Input: part model. Units: mm. Frame: model coordinates. A direction names the side the tool comes from. Give positions to 0.01 mm unless a question says otherwise; leave off trailing zeros. Loops run counter-clockwise (first coordinate to the right, second up) from the corner with the lowest first, then second, coordinate; pieces in that order, holes last. Notation, with made-up numbers: (-30, 7.5) - (12, 7.5) arc R28 ccw to (12, 37.5) - close; hole circle Ø1 at (-7, 6.5). An arc over 180 degrees is marked (long way). Answer as a JSON object with one key per item and string values.
Autodesk Inventor part; units mm, degrees
ref_plane "YZ Plane" through (0, 0, 0) normal (1, 0, 0) x (0, 1, 0)
ref_plane "XZ Plane" through (0, 0, 0) normal (0, 1, 0) x (-1, 0, 0)
ref_plane "XY Plane" through (0, 0, 0) normal (0, 0, 1) x (1, 0, 0)
sketch "Sketch1" plane through (0, 0, 0) normal (1, 0, 0) x (0, 1, 0)
  circle A0 centre (0, 0) radius 35
  line L0 (29.5804, -5) -> (4.8166, -1.3417)
  line L1 (36.6755, 0) -> (35, 0)
  line L2 (29.5804, 5) -> (4.8166, 1.3417)
  line L3 (17.381, 24.452) -> (2.4572, 4.3546)
  line L4 (24.452, 17.381) -> (4.3546, 2.4572)
  line L5 (-5, 29.5804) -> (-1.3417, 4.8166)
  line L6 (5, 29.5804) -> (1.3417, 4.8166)
  line L7 (-24.452, 17.381) -> (-4.3546, 2.4572)
  line L8 (-17.381, 24.452) -> (-2.4572, 4.3546)
  line L9 (-29.5804, -5) -> (-4.8166, -1.3417)
  line L10 (-29.5804, 5) -> (-4.8166, 1.3417)
  line L11 (-17.381, -24.452) -> (-2.4572, -4.3546)
  line L12 (-24.452, -17.381) -> (-4.3546, -2.4572)
  line L13 (5, -29.5804) -> (1.3417, -4.8166)
  line L14 (-5, -29.5804) -> (-1.3417, -4.8166)
  line L15 (24.452, -17.381) -> (4.3546, -2.4572)
  line L16 (17.381, -24.452) -> (2.4572, -4.3546)
  arc A1 (4.8166, 1.3417) -> (4.3546, 2.4572) centre (0, 0) ccw
  arc A2 (2.4572, 4.3546) -> (1.3417, 4.8166) centre (0, 0) ccw
  arc A3 (-1.3417, 4.8166) -> (-2.4572, 4.3546) centre (0, 0) ccw
  arc A4 (-4.3546, 2.4572) -> (-4.8166, 1.3417) centre (0, 0) ccw
  arc A5 (-4.8166, -1.3417) -> (-4.3546, -2.4572) centre (0, 0) ccw
  arc A6 (-2.4572, -4.3546) -> (-1.3417, -4.8166) centre (0, 0) ccw
  arc A7 (1.3417, -4.8166) -> (2.4572, -4.3546) centre (0, 0) ccw
  arc A8 (4.3546, -2.4572) -> (4.8166, -1.3417) centre (0, 0) ccw
  arc A9 (29.5804, 5) -> (24.452, 17.381) centre (0, 0) ccw
  arc A10 (24.452, -17.381) -> (29.5804, -5) centre (0, 0) ccw
  arc A11 (5, -29.5804) -> (17.381, -24.452) centre (0, 0) ccw
  arc A12 (-17.381, -24.452) -> (-5, -29.5804) centre (0, 0) ccw
  arc A13 (-29.5804, -5) -> (-24.452, -17.381) centre (0, 0) ccw
  arc A14 (-24.452, 17.381) -> (-29.5804, 5) centre (0, 0) ccw
  arc A15 (17.381, 24.452) -> (5, 29.5804) centre (0, 0) ccw
  arc A16 (-5, 29.5804) -> (-17.381, 24.452) centre (0, 0) ccw
  dimension "d0" = 70
extrude "Extrusion1" add sketch "Sketch1" along normal blind 8
sketch "Sketch2" plane through (8, 0, 0) normal (1, 0, 0) x (0, 0, -1)
  circle A0 centre (0, 0) radius 30
  dimension "d9" = 60
extrude "Extrusion2" cut sketch "Sketch2" against normal blind 1
sketch "Sketch3" plane through (0, 0, 0) normal (-1, 0, 0) x (0, 0, 1)
  circle A0 centre (0, 0) radius 30
extrude "Extrusion3" cut sketch "Sketch3" against normal blind 1
fillet "Fillet1" radius 2 2 edges at (0, -35, 0) (8, -35, 0)
sketch "Sketch4" plane through (1, 0, 0) normal (-1, 0, 0) x (0, 0, 1)
  circle A0 centre (0, 0) radius 1.5
  dimension "d15" = 3
extrude "Extrusion4" cut sketch "Sketch4" against normal blind 10
properties part number "Wheel"
Item 1: Cut plane A-A (z = 0). Return loops of the section in (x, y).
Geometry check:
{"outline": "(0, -33) arc R2 ccw to (2, -35) - (6, -35) arc R2 ccw to (8, -33) - (8, -30) - (7, -30) - (7, -1.5) - (1, -1.5) - (1, -30) - (0, -30) - close; (0, 30) - (1, 30) - (1, 1.5) - (7, 1.5) - (7, 30) - (8, 30) - (8, 33) arc R2 ccw to (6, 35) - (2, 35) arc R2 ccw to (0, 33) - close"}
Item 2: Contact query for flat-ended pins moving along their axis: P1, Ø8, axis at y = 0, z = 16, coming from the +X side; P2, Ø1, axis at x = 2, y = 24.5, coming from the +Z side; P3, Ø1, axis at x = 6, y = -27.5, coming from the -Z side. Output: stop coordinate, or through.
Geometry check:
{"P1": "stops at x = 7", "P2": "stops at z = 25.48", "P3": "stops at z = -22.27"}
Item 3: Access query for faces 1 (the face through (0.493, -21.163, -21.263)), 2 (the face through (3.96, -10.02, -14.54)), 3 (the face through (7.507, -21.263, -21.163)). Directions: +Z, -Z, +X, -X, +Y, -Y. A direction counts if a zero-diameter tool reaches every point of the face in a straight line with its end or side. Return the directions, or none.
Geometry check:
{"face 1": "-X", "face 2": "+X, -X", "face 3": "+X"}
Item 4: Material intervals for line 1 (Z direction, x = 5, y = -25.5); line 2 (Z direction, x = 3, y = 25); line 3 (X direction, y = 23, z = 17), sorted ascending. Write a range as [from, to].
Geometry check:
{"line 1": "z = [-23.97, -15.8], [-4.4, 4.4], [15.8, 23.97]", "line 2": "z = [-24.49, -16.58], [-4.32, 4.32], [16.58, 24.49]", "line 3": "x = [1, 7]"}
Item 5: Mould query, pull axis Z, two halves, no side actions, for faces 4 (the face through (0, 15, -27)), 5 (the face through (4, -28, 21)), 6 (the face through (7.507, -21.163, 21.263)). Classes: released by +Z, released by -Z, zero draft, split by the parting line, or undercut.
Geometry check:
{"face 4": "zero draft", "face 5": "split by the parting line", "face 6": "undercut"}
Item 6: Cut plane C-C (x = 3.75). Give the number of separate pieces and of enclosed holes in the cut face, then the cut area to 3 significant figures.
Geometry check:
{"separate pieces": "1", "enclosed holes": "9", "area": "2,370 mm2"}
